from build123d import *

# Parameters (mm, degrees)
BOSS_EXTRUDE1_DEPTH         = 25.4
F_1_4_CLEARANCE_HOLE1_D     = 6.7564
F_1_4_CLEARANCE_HOLE1_DEPTH = 10.16
F_1_4_CLEARANCE_HOLE1_TIP   = 2.029827343
F_1_4_CLEARANCE_HOLE2_D     = 6.7564
F_1_4_CLEARANCE_HOLE2_DEPTH = 10.16
F_1_4_CLEARANCE_HOLE2_TIP   = 2.029827343
SKETCH8_R                   = 5.715
CUT_EXTRUDE1_DEPTH          = 5.08
SKETCH9_R                   = 5.715
CUT_EXTRUDE2_DEPTH          = 5.08


with BuildPart() as part:
    # Sketch1 → Boss-Extrude1 (new body)
    with BuildSketch(Plane.XY):
        Polygon((10.16, 0), (0, 0), (0, 54.048005464), (83.514454911, 15.104575572), (79.220653372, 5.896488455), (10.16, 38.1), align=None)
    extrude(amount=BOSS_EXTRUDE1_DEPTH)

    # 1/4 Clearance Hole1
    with Locations(Plane.ZY):
        with Locations((12.7, 12.7)):
            Hole(F_1_4_CLEARANCE_HOLE1_D / 2, depth=F_1_4_CLEARANCE_HOLE1_DEPTH)
            with Locations((0, 0, -(F_1_4_CLEARANCE_HOLE1_DEPTH + F_1_4_CLEARANCE_HOLE1_TIP / 2))):  # 118° drill point
                Cone(0, F_1_4_CLEARANCE_HOLE1_D / 2, F_1_4_CLEARANCE_HOLE1_TIP, mode=Mode.SUBTRACT)

    # 1/4 Clearance Hole2
    with Locations(Plane(origin=(20.701587123, 44.394696852, 0), x_dir=(0.9063077870366483, -0.42261826174070316, 0), z_dir=(0.42261826174070316, 0.9063077870366483, 0))):
        with Locations((56.606331344, -12.7)):
            Hole(F_1_4_CLEARANCE_HOLE2_D / 2, depth=F_1_4_CLEARANCE_HOLE2_DEPTH)
            with Locations((0, 0, -(F_1_4_CLEARANCE_HOLE2_DEPTH + F_1_4_CLEARANCE_HOLE2_TIP / 2))):  # 118° drill point
                Cone(0, F_1_4_CLEARANCE_HOLE2_D / 2, F_1_4_CLEARANCE_HOLE2_TIP, mode=Mode.SUBTRACT)

    # Fillet1
    # a fillet whose section is not a circle: 5.08 mm, written as the material it adds along each edge (its section moved 0.00015 mm through the faces so that the kernel can cut it)
    with BuildSketch(Plane(origin=(10.16, 38.1, 0), x_dir=(0.9063157368032501, -0.4226012129925586, 0), z_dir=(0, 0, 1))) as fillet1_piece_1:
        with BuildLine():
            add(Edge.make_bspline([(7.974002733, 0), (6.748845081, 2.3047e-05), (5.523687428, 4.6093e-05), (2.911264627, -0.681700719), (1.848095837, -2.35047216), (2.334181059, -5.00626823), (2.851934169, -6.11664789), (3.369687279, -7.227027551)], knots=[0, 0, 0, 0, 0, 0, 0.5, 0.5, 1, 1, 1, 1, 1, 1], degree=5))
            Line((3.369687279, -7.227027551), (3.277605601, -7.269963835))
            ThreePointArc((3.277605601, -7.269963835), (1.592829935, -3.656418364), (-0.092081679, -0.042936283))
            Line((-0.092081679, -0.042936283), (1.911e-06, 0.1016))
            ThreePointArc((1.911e-06, 0.1016), (3.987003276, 0.101525), (7.974004644, 0.1016))
            Line((7.974004644, 0.1016), (7.974002733, 0))
        make_face()
    extrude(amount=25.4)
    # a fillet whose section is not a circle: 5.08 mm, written as the material it takes off along each edge (its section moved 0.00015 mm through the faces so that the kernel can cut it)
    with BuildSketch(Plane(origin=(0, 54.048005464, -19.935006833), x_dir=(-1.8811129744924416e-05, -0.9999999998230706, 0), z_dir=(0, 0, 1))) as fillet1_2_piece_1:
        with BuildLine():
            add(Edge.make_bspline([(7.974002733, 0), (6.748845081, -2.3047e-05), (5.523687428, -4.6093e-05), (2.911264627, 0.681700719), (1.848095837, 2.35047216), (2.334181059, 5.00626823), (2.851934169, 6.11664789), (3.369687279, 7.227027551)], knots=[0, 0, 0, 0, 0, 0, 0.5, 0.5, 1, 1, 1, 1, 1, 1], degree=5))
            Line((3.369687279, 7.227027551), (3.277605601, 7.269963835))
            ThreePointArc((3.277605601, 7.269963835), (1.592829935, 3.656418364), (-0.092081679, 0.042936283))
            Line((-0.092081679, 0.042936283), (1.911e-06, -0.1016))
            ThreePointArc((1.911e-06, -0.1016), (3.987003276, -0.101525), (7.974004644, -0.1016))
            Line((7.974004644, -0.1016), (7.974002733, 0))
        make_face()
    extrude(amount=65.270013666, mode=Mode.SUBTRACT)

    # Sketch8 → Cut-Extrude1 (cut)
    with BuildSketch(Plane(origin=(16.407785584, 35.186609736, 0), x_dir=(0.906307787036648, -0.42261826174070366, 0), z_dir=(-0.4226182617407036, -0.9063077870366479, 0))):
        with Locations((56.606331344, 12.7)):
            Circle(SKETCH8_R)
    extrude(amount=-CUT_EXTRUDE1_DEPTH, mode=Mode.SUBTRACT)

    # Sketch9 → Cut-Extrude2 (cut)
    with BuildSketch(Plane(origin=(10.16, 0, 0), x_dir=(0, 0, -1), z_dir=(1, 0, 0))):
        with Locations(Location((-12.7, 12.7, 0), (0, 0, 90))):
            Circle(SKETCH9_R)
    extrude(amount=-CUT_EXTRUDE2_DEPTH, mode=Mode.SUBTRACT)


solid = part.part
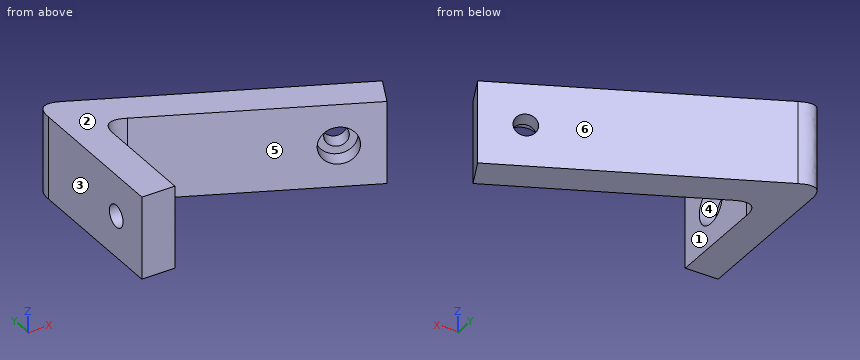
Geometry: final body of the model. Coordinates: model frame, mm. Face numbers are marked on the shaded views. A direction names the side the tool comes from. Give positions to 0.01 mm unless a question says otherwise; leave off trailing zeros. Order: outer loops, then holes, each group sorted by start corner. A loop starts at its lowest first (then second) coordinate and runs counter-clockwise, first axis right, second up. Notation, with made-up numbers: (-37.5, 81) -> (9.5, 81) arc R20 ccw to (9.5, 113) -> close; hole circle Ø5 at (52, 2.5). An arc over 180 degrees is marked (long way). Answer as a JSON object with one key per item and string values.
Q1. Section C-C (y = 38). Output: boundary loops of the cut face in (x, z).
Entries:
{"outline": "(0, 0) -> (34.42, 0) -> (34.42, 25.4) -> (0, 25.4) -> close"}
Q2. Material intervals for probe 1 along Z at (x, y) = (8.1, 12.7) (3 decimals); probe 2 along X at (y, z) = (27, 8.5); probe 3 along X at (y, z) = (23.5, 17.25), sorted ascending.
Entries:
{"probe 1": "z = 0 to 6.985, 18.415 to 25.4", "probe 2": "x = 0 to 10.16, 33.96 to 58", "probe 3": "x = 0 to 10.16, 41.47 to 65.51"}
Q3. First-contact query: pin 1 (5 mm diameter, centred on y = 31.5, z = 18, fed in from +X); pin 2 (5 mm diameter, centred on x = 44, z = 8.5, fed in from +Y); pin 3 (8 mm diameter, centred on y = 43, z = 16, fed in from +X); pin 4 (10 mm diameter, centred on x = 58.5, y = 8.5, fed in from +Z). Flat tips, straight axial feed; report the tip coordinate or a pass-through.
Entries:
{"pin 1": "stops at x = 53.72", "pin 2": "stops at y = 34.7", "pin 3": "stops at x = 32.27", "pin 4": "passes through"}
Q4. Section B-B (x = 41.5). Output: boundary loops of the cut face in (y, z), plus the area to 3 significant figures.
Entries:
{"outline": "(23.49, 0) -> (34.7, 0) -> (34.7, 25.4) -> (23.49, 25.4) -> close", "area": "285 mm^2"}
Q5. Section A-A (z = 12.7). State how many separate pieces and enclosed holes the cut face has, plus the area to 3 significant figures.
Entries:
{"separate pieces": "3", "enclosed holes": "0", "area": "1,140 mm^2"}
Q6. Draft query along X for the marked faces 1, 2 and 3. Return one class per face: released by +X, released by -X, zero draft, split by the parting line, or undercut.
Entries:
{"face 1": "undercut", "face 2": "zero draft", "face 3": "released by -X"}
Q7. Access query for the marked faces 4, 5 and 6. Directions: +Z, -Z, +X, -X, +Y, -Y. A direction counts if a zero-diameter tool reaches every point of the face in a straight line with its end or side. Return the directions, or none.
Entries:
{"face 4": "none", "face 5": "+Z, -Z, -Y", "face 6": "+Z, -Z, +X, +Y"}
